Here's how the part is built. I have some questions about the finished solid (model axes, mm). A direction names the side the tool comes from. Round coordinates to 2 decimals unless told otherwise and drop trailing zeros. Loops run counter-clockwise (first coordinate to the right, second up) from the corner with the lowest first, then second, coordinate; pieces in that order, holes last. Notation, with made-up numbers: M 29.25,65.25 L 84.25,65.25 A28 cw 84.25,89.25 Z; hole C 21,50.25 d6. An arc over 180 degrees is marked long. Answer as a JSON object with one key per item and string values.
from build123d import *

# Parameters (mm, degrees)
BASPROSKE_W             = 4
BASPROSKE_H             = 11
TOOTHCUT_DEPTH          = 17.062378404
TEETHCUTS_COUNT         = 20
TEETHCUTS_ANGLE         = 342
BORSKE_R                = 2.5
BORE_DEPTH              = 50.0000508
SKETCH2_R               = 5
BOSS_EXTRUDE2_DEPTH     = 15
SKETCH3_R               = 8.5
BOSS_EXTRUDE3_DEPTH     = 3
SKETCH4_R               = 2.65
CUT_EXTRUDE1_DEPTH      = 27.864619954
CUT_EXTRUDE1_DEPTH_BACK = 27.864619954


with BuildPart() as part:
    # BasProSke → Base-Revolve (revolve)
    with BuildSketch(Plane(origin=(0, 0, 0), x_dir=(1, 0, 0), z_dir=(0, 1, 0)), mode=Mode.PRIVATE) as base_revolve_sk:
        with Locations((2, 5.5)):
            Rectangle(BASPROSKE_W, BASPROSKE_H)
    revolve(base_revolve_sk.sketch.rotate(Axis((-10, 0, 0), (1, 0, 0)), 180), axis=Axis((-10, 0, 0), (1, 0, 0)))

    # TooCutSke → ToothCut (cut, through all)
    with BuildSketch(Plane(origin=(0, 0, 0), x_dir=(0, 0, -1), z_dir=(1, 0, 0))):
        with BuildLine():
            ThreePointArc((0.499924007, 8.734705318), (0, 8.749), (-0.499924007, 8.734705318))
            ThreePointArc((-0.499924007, 8.734705318), (-0.824302243, 9.905497836), (-1.485192705, 10.924909509))
            ThreePointArc((-1.485192705, 10.924909509), (0, 11.0254), (1.485192705, 10.924909509))
            ThreePointArc((1.485192705, 10.924909509), (0.824302243, 9.905497836), (0.499924007, 8.734705318))
        make_face()
    toothcut = extrude(amount=TOOTHCUT_DEPTH, mode=Mode.SUBTRACT)

    # TeethCuts: ToothCut ×20 about axis
    teethcuts_axis = Axis((-10, 0, 0), (1, 0, 0))
    for i in range(1, TEETHCUTS_COUNT):
        add(toothcut.rotate(teethcuts_axis, i * TEETHCUTS_ANGLE / (TEETHCUTS_COUNT - 1)), mode=Mode.SUBTRACT)

    # BorSke → Bore (cut, symmetric)
    with BuildSketch(Plane(origin=(0, 0, 0), x_dir=(0, 0, -1), z_dir=(1, 0, 0))):
        with Locations(Location((0, 0, 0), (0, 0, 180))):
            Circle(BORSKE_R)
    extrude(amount=BORE_DEPTH, both=True, mode=Mode.SUBTRACT)

    # Sketch2 → Boss-Extrude2 (add)
    with BuildSketch(Plane(origin=(4, 0, 0), x_dir=(0, 0, -1), z_dir=(1, 0, 0))):
        with Locations(Location((0, 0, 0), (0, 0, 180))):
            Circle(SKETCH2_R)
    extrude(amount=BOSS_EXTRUDE2_DEPTH)

    # Sketch3 → Boss-Extrude3 (add)
    with BuildSketch(Plane(origin=(19, 0, 0), x_dir=(0, 0, -1), z_dir=(1, 0, 0))):
        Circle(SKETCH3_R)
    extrude(amount=BOSS_EXTRUDE3_DEPTH)

    # Sketch4 → Cut-Extrude1 (cut, two sides)
    with BuildSketch(Plane(origin=(22, 0, 0), x_dir=(0, 0, -1), z_dir=(1, 0, 0))) as cut_extrude1_sk:
        with Locations(Location((0, 0, 0), (0, 0, 180))):
            Circle(SKETCH4_R)
    extrude(amount=CUT_EXTRUDE1_DEPTH, mode=Mode.SUBTRACT)
    extrude(cut_extrude1_sk.sketch, amount=-CUT_EXTRUDE1_DEPTH_BACK, mode=Mode.SUBTRACT)


solid = part.part
Item 1: I want a section at C-C on x = 13. List the corners of the cut face in (y, z) for me, plus the area to 3 significant figures.
Solution:
{"outline": "C 0,0 d10; hole C 0,0 d5.3", "area": "56.5 mm2"}
Item 2: I want a section at A-A on y = 0. List the corners of the cut face in (x, z) for me.
Solution:
{"outline": "M 0,-8.75 L 4,-8.75 L 4,-5 L 19,-5 L 19,-8.5 L 22,-8.5 L 22,-2.65 L 0,-2.65 Z; M 0,2.65 L 22,2.65 L 22,8.5 L 19,8.5 L 19,5 L 4,5 L 4,8.75 L 0,8.75 Z"}
Item 3: We'd pull the mould along X, two halves only. Please class faces 1 (the face through (22, 2, -2)), 2 (the face through (4, 2, -5)), 3 (the face through (1.972, 2.277, -9.677)): +X half, -X half, draft (parallel to the pull), parting line (faces both ways), or undercut.
Solution:
{"face 1": "+X half", "face 2": "undercut", "face 3": "draft"}
Item 4: I want a section at D-D on y = -4. List the corners of the cut face in (x, z) for me, plus the area to 3 significant figures.
Solution:
{"outline": "M 0,-9.33 L 4,-9.33 L 4,-3 L 19,-3 L 19,-7.5 L 22,-7.5 L 22,7.5 L 19,7.5 L 19,3 L 4,3 L 4,9.33 L 0,9.33 Z", "area": "210 mm2"}
Item 5: For faces 4 (the face through (1.97, -9.17, 3.85)), 5 (the face through (1.972, 5.148, 7.074)), 6 (the face through (1.972, -6.461, 7.513)), which set-ups out of +Z, -Z, +X, -X, +Y, -Y let a thin tool reach every point of the face, with its end or its side?
Solution:
{"face 4": "+X, -X, -Y", "face 5": "+X, -X", "face 6": "+Z, +X, -X"}
Item 6: If I drill on L1, parallel to X at y = 5.25, z = -0.25; L2, parallel to Y at x = 12, z = 0; L3, parallel to Y at x = 6, z = -1.25, over which ranges is the centre line in solid material (lowest first)? Write a range as from..to.
Solution:
{"L1": "x = 0..4, 19..22", "L2": "y = -5..-2.65, 2.65..5", "L3": "y = -4.84..-2.34, 2.34..4.84"}
Item 7: For P1, Ø4, axis at x = 12, y = 3.5, coming from the -Z side; P2, Ø5, axis at x = 3.5, y = -7.5, coming from the +Z side; P3, Ø1, axis at x = 12, z = 2.5, coming from the +Y side, each with a flat end and sliding along its axis, tell me the tip position at first contact or that it passes through.
Solution:
{"P1": "stops at z = -4.77", "P2": "stops at z = 9.8", "P3": "stops at y = 4.58"}
